For this review, take the finished solid that the model builds, in its own axes (mm). A direction names the side the tool comes from. Give positions to 0.01 mm unless a question says otherwise; leave off trailing zeros. Write each loop counter-clockwise with the first axis right and the second up, starting at its lowest first coordinate (ties: lowest second). Pieces come first, ordered by that corner, then holes.
1) For P1, Ø2, axis at x = -68.5, z = 2.5, coming from the +Y side, flat-tipped, find the tip position at first contact; note if it passes through.
2) We need section D-D on x = -75. Give the boundary of the cut face in (y, z).
3) We need section C-C on x = -60. Give the boundary of the cut face in (y, z), and give its area (3 significant figures).
4) We need section A-A on y = 39. Give the boundary of the cut face in (x, z), and give its area (3 significant figures).
5) Draft analysis for pull direction Y (two halves, no side actions). For faces 1 (the face through (-61, 32, 0)), 2 (the face through (-71.71, 52.947, 1.972)), 3 (the face through (-74.194, 65.265, 1.972)), state which applies: pulls with the +Y half, pulls with the -Y half, needs draft (parallel to the pull), parting line crosses it, or undercut.
6) Wall thickness on line 1 along Y through (x, z) = (-57.5, 3.3); line 2 along Y through (x, z) = (-63, 3.6); line 3 along Y through (x, z) = (-60, 2.7): over which ranges is each line inside the solid? List them lowest first.
7) We need section B-B on z = 1.25. Give the boundary of the cut face in (x, y).
8) Machinability: for faces 4 (the face through (-65, 21, 2)), 5 (the face through (-59.077, 46.226, 1.972)), which of the approach directions +Z, -Z, +X, -X, +Y, -Y give a long, thin tool a straight path to every point of the face, cutting with its end or side? Answer none if there is none.
from build123d import *

# Parameters (mm, degrees)
SKETCH_2_R      = 3.6
SKETCH_2_R_2    = 1.5
SKETCH_2_R_3    = 2
EXTRUDE_1_DEPTH = 4
FILLET_1_R      = 2


with BuildPart() as part:
    # 草图2 → 凸台-拉伸1 (new body)
    with BuildSketch(Plane.XY):
        with BuildLine():
            Line((-65, 0), (-65, 44))
            Line((-65, 44), (-78.2, 61.6))
            ThreePointArc((-78.2, 61.6), (-77.728789328, 66.924672427), (-72.384272007, 67.026213321))
            Line((-72.384272007, 67.026213321), (-55, 52))
            Line((-55, 52), (-55, 0))
            ThreePointArc((-55, 0), (-60, -5), (-65, 0))
        make_face()
        with Locations((-60, 39)):
            Circle(SKETCH_2_R, mode=Mode.SUBTRACT)
        with Locations((-60, 0)):
            Circle(SKETCH_2_R, mode=Mode.SUBTRACT)
        with Locations((-75, 64)):
            Circle(SKETCH_2_R_2, mode=Mode.SUBTRACT)
        with Locations((-60, 19.75)):
            Circle(SKETCH_2_R_3, mode=Mode.SUBTRACT)
        with Locations((-60, 48)):
            Circle(SKETCH_2_R_3, mode=Mode.SUBTRACT)
    extrude(amount=EXTRUDE_1_DEPTH)

    # 圆角1
    fillet_1_edges = [part.edges().sort_by_distance(p)[0] for p in [
        (-55, 52, 2),
        (-65, 44, 2),
    ]]
    fillet(fillet_1_edges, radius=FILLET_1_R)


solid = part.part
Results list:
1. P1: stops at y = 64.53
2. outline: (57.33, 0) - (62.5, 0) - (62.5, 4) - (57.33, 4) - close; (65.5, 0) - (68, 0) - (68, 4) - (65.5, 4) - close
3. outline: (-5, 0) - (-3.6, 0) - (-3.6, 4) - (-5, 4) - close; (3.6, 0) - (17.75, 0) - (17.75, 4) - (3.6, 4) - close; (21.75, 0) - (35.4, 0) - (35.4, 4) - (21.75, 4) - close; (42.6, 0) - (46, 0) - (46, 4) - (42.6, 4) - close; (50, 0) - (56.32, 0) - (56.32, 4) - (50, 4) - close
3. area: 156 mm2
4. outline: (-65, 0) - (-63.6, 0) - (-63.6, 4) - (-65, 4) - close; (-56.4, 0) - (-55, 0) - (-55, 4) - (-56.4, 4) - close
4. area: 11.2 mm2
5. face 1: needs draft
5. face 2: pulls with the -Y half
5. face 3: undercut
6. line 1: y = -4.33 to -2.59, 2.59 to 36.41, 41.59 to 54.16
6. line 2: y = -4 to -1.99, 1.99 to 37.01, 40.99 to 58.91
6. line 3: y = -5 to -3.6, 3.6 to 17.75, 21.75 to 35.4, 42.6 to 46, 50 to 56.32
7. outline: (-78.2, 61.6) - (-65.4, 44.53) arc R2 cw to (-65, 43.33) - (-65, 0) arc R5 ccw to (-55, 0) - (-55, 51.09) arc R2 ccw to (-55.69, 52.6) - (-72.38, 67.03) arc R4 ccw to start; hole circle Ø3 at (-75, 64); hole circle Ø7.2 at (-60, 0); hole circle Ø7.2 at (-60, 39); hole circle Ø4 at (-60, 19.75); hole circle Ø4 at (-60, 48)
8. face 4: +Z, -Z, -X, -Y
8. face 5: +Z, -Z
